Verification items for the finished model (mm, model axes). Coordinates: 2 decimals unless noted, no trailing zeros. Write each loop counter-clockwise with the first axis right and the second up, starting at its lowest first coordinate (ties: lowest second). Pieces come first, ordered by that corner, then holes. Notation, with made-up numbers: (-6.5, 47.25) - (32.5, 47.25) arc R19 cw to (32.5, 84.25) - close; hole circle Ø2 at (61.25, -38). An arc over 180 degrees is marked (long way). Use one line per item in the form item = value. Start each with the question number.
(1) Sectioned sample at B-B (z = -2). Record the cut outline in (x, y), and give its area (3 significant figures).
(2) Material ranges on line 1 (Y direction, x = -1.5, z = -4); line 2 (Z direction, x = -0.25, y = 55); line 3 (X direction, y = 67, z = -0.25), recorded low to high. Write a range as [from, to].
(3) Mould release check, pull along Y, two halves, no side actions. Record for faces 1 (the cylindrical face through (3.905, 43.306, -0.867)), 2 (the cylindrical face through (-4.88, 54.89, -1.08)), 3 (the flat face through (0, 115, 0)), 4 (the cylindrical face through (3.905, 66.806, -0.867)): released by +Y, released by -Y, zero draft, split by the parting line, or undercut.
(4) Sectioned sample at A-A (x = -1.5). Record the cut outline in (y, z).
(5) Gauge pin test, flat ends, axial feed: pin 1 Ø3 at (x, y) = (2, 22) entering from -Z; pin 2 Ø1.5 at (y, z) = (35.5, -1.5) entering from +X. Record the tip position at first contact, or that the pin passes through.
(6) Sectioned sample at C-C (y = 10.5). Record the cut outline in (x, z), and give its area (3 significant figures).
from build123d import *

# Parameters (mm, degrees)
SKETCH1_R           = 5
BOSS_EXTRUDE1_DEPTH = 115
SKETCH2_W           = 1
SKETCH2_H           = 0.8
LPATTERN1_COUNT     = 2
LPATTERN1_PITCH     = 23.5


with BuildPart() as part:
    # Sketch1 → Boss-Extrude1 (new body)
    with BuildSketch(Plane(origin=(0, 0, 0), x_dir=(1, 0, 0), z_dir=(0, 1, 0))):
        with Locations(Location((0, 0, 0), (0, 0, 270))):
            Circle(SKETCH1_R)
    extrude(amount=BOSS_EXTRUDE1_DEPTH)

    # Sketch2 → Cut-Revolve1 (revolve, cut)
    with BuildSketch(Plane(origin=(0, 0, 0), x_dir=(0, 0, -1), z_dir=(1, 0, 0)), mode=Mode.PRIVATE) as cut_revolve1_sk:
        with Locations((4.5, 66.8)):
            Rectangle(SKETCH2_W, SKETCH2_H)
    cut_revolve1 = revolve(cut_revolve1_sk.sketch.rotate(Axis((0, 115, 0), (0, -1, 0)), 180), axis=Axis((0, 115, 0), (0, -1, 0)), mode=Mode.SUBTRACT)

    # LPattern1: Cut-Revolve1 ×2
    with Locations(*[(0, -i * LPATTERN1_PITCH, 0) for i in range(1, LPATTERN1_COUNT)]):
        add(cut_revolve1, mode=Mode.SUBTRACT)


solid = part.part
Answers below:
q1.outline = (-4.58, 0) - (4.58, 0) - (4.58, 42.9) - (3.46, 42.9) - (3.46, 43.7) - (4.58, 43.7) - (4.58, 66.4) - (3.46, 66.4) - (3.46, 67.2) - (4.58, 67.2) - (4.58, 115) - (-4.58, 115) - (-4.58, 67.2) - (-3.46, 67.2) - (-3.46, 66.4) - (-4.58, 66.4) - (-4.58, 43.7) - (-3.46, 43.7) - (-3.46, 42.9) - (-4.58, 42.9) - close
q1.area = 1,050 mm2
q2.line_1 = [0, 42.9], [43.7, 66.4], [67.2, 115]
q2.line_2 = [-4.99, 4.99]
q2.line_3 = [-3.99, 3.99]
q3.face_1 = undercut
q3.face_2 = zero draft
q3.face_3 = released by +Y
q3.face_4 = undercut
q4.outline = (0, -4.77) - (42.9, -4.77) - (42.9, -3.71) - (43.7, -3.71) - (43.7, -4.77) - (66.4, -4.77) - (66.4, -3.71) - (67.2, -3.71) - (67.2, -4.77) - (115, -4.77) - (115, 4.77) - (67.2, 4.77) - (67.2, 3.71) - (66.4, 3.71) - (66.4, 4.77) - (43.7, 4.77) - (43.7, 3.71) - (42.9, 3.71) - (42.9, 4.77) - (0, 4.77) - close
q5.pin_1 = -4.97
q5.pin_2 = 4.94
q6.outline = circle Ø10 at (0, 0)
q6.area = 78.5 mm2
